Autodesk Inventor part; units mm, degrees
ref_plane "YZ Plane" through (0, 0, 0) normal (1, 0, 0) x (0, 1, 0)
ref_plane "XZ Plane" through (0, 0, 0) normal (0, 1, 0) x (-1, 0, 0)
ref_plane "XY Plane" through (0, 0, 0) normal (0, 0, 1) x (1, 0, 0)
sketch "Sketch1" plane through (0, 0, 0) normal (0, 1, 0) x (-1, 0, 0)
  line L0 (0, 0) -> (10, 0)
  line L1 (10, 0) -> (10, -12.7)
  line L2 (10, -12.7) -> (0, -12.7)
  line L3 (0, -12.7) -> (0, 0)
  dimension "d0" = 10
  dimension "d1" = 12.7
extrude "Extrusion1" add sketch "Sketch1" along normal blind 5.6
sketch "Sketch2" plane through (-10, 0, -12.7) normal (-1, 0, 0) x (0, 0, 1)
  line L0 (3.3, 4.8) -> (9.4, 4.8)
  line L1 (9.4, 4.8) -> (9.4, 0.8)
  line L2 (9.4, 0.8) -> (3.3, 0.8)
  line L3 (3.3, 0.8) -> (3.3, 4.8)
  line L4 (0, 0) -> (0, 5.6)
  point P0 (12.7, 0)
  point P1 (6.35, 4.8)
  point P2 (9.4, 2.8)
  dimension "d4" = 6.1
  dimension "d5" = 4
  dimension "d6" = 2.8
  dimension "d7" = 6.35
extrude "Extrusion2" cut sketch "Sketch2" against normal blind 1
sketch "Sketch3" plane through (-9, 0, -12.7) normal (-1, 0, 0) x (0, 0, 1)
  line L0 (5.8365, 4.7365) -> (9.3365, 4.7365)
  line L1 (9.3365, 4.7365) -> (9.3365, 0.8765)
  line L2 (9.3365, 0.8765) -> (5.8365, 0.8765)
  line L3 (5.8365, 0.8765) -> (5.8365, 4.7365)
  line L4 (9.4, 4.8) -> (9.4, 0.8)
  line L5 (3.3, 4.8) -> (9.4, 4.8)
  point P0 (12.7, 0)
  dimension "d10" = 3.5
  dimension "d11" = 3.86
  dimension "d12" = 0.0635
  dimension "d13" = 0.0635
extrude "Extrusion3" add sketch "Sketch3" along normal blind 5.72
properties part number "103-5007-EV"
Can you work these out from the model? Positions are in its coordinate system, mm. A direction names the side the tool comes from. Coordinates: 2 decimals unless noted, no trailing zeros. Order: outer loops, then holes, each group sorted by start corner. A loop starts at its lowest first (then second) coordinate and runs counter-clockwise, first axis right, second up.
1. I need wall thicknesses on line 1 (Y direction, x = -14, z = -6); line 2 (X direction, y = 3.9, z = -12); line 3 (Z direction, x = -11, y = 3.65). Which ranges of each line are inside material? Lowest first, please.
2. If we section it at D-D (x = -11): Please give me the cut outline in (y, z).
3. For faces 5 (the face through (-12, 4.736, -5)), 6 (the face through (0, 3, -6)), which set-ups out of +Z, -Z, +X, -X, +Y, -Y let a thin tool reach every point of the face, with its end or its side?
4. If we section it at C-C (z = -6): Please give me the cut outline in (x, y).
5. I'm going to push flat-ended pins straight in: pin 1 (0.5 mm diameter, centred on x = -9.5, y = 3.5, fed in from +Z); pin 2 (2 mm diameter, centred on x = -11.5, y = 3, fed in from +Z); pin 3 (1 mm diameter, centred on x = -12, z = -4.5, fed in from +Y); pin 4 (3 mm diameter, centred on y = 2.5, z = -10.5, fed in from -X). Where does each tip first touch, or does it pass through?
6. If we section it at A-A (x = -9.25): Please give me the cut outline in (y, z).
7. If we section it at B-B (y = 4.55): Please give me the cut outline in (x, z).
8. Thinking about a two-plate mould opening in Z: for faces 1 (the face through (-9, 3, -8)), 2 (the face through (-14.72, 3, -5)), 3 (the face through (-9.5, 2.8, -9.4)), 4 (the face through (-5, 3, 0)), which applies, +Z half, -Z half, draft (parallel to the pull), parting line (faces both ways), or undercut?
Entries:
1. line 1: y = 0.88 to 4.74
1. line 2: x = -10 to 0
1. line 3: z = -6.86 to -3.36
2. outline: (0.88, -6.86) - (4.74, -6.86) - (4.74, -3.36) - (0.88, -3.36) - close
3. face 5: -X
3. face 6: +Z, -Z, +X, +Y, -Y
4. outline: (-14.72, 0.88) - (-9, 0.88) - (-9, 0.8) - (-10, 0.8) - (-10, 0) - (0, 0) - (0, 5.6) - (-10, 5.6) - (-10, 4.8) - (-9, 4.8) - (-9, 4.74) - (-14.72, 4.74) - close
5. pin 1: stops at z = 0
5. pin 2: stops at z = -3.36
5. pin 3: stops at y = 4.74
5. pin 4: stops at x = -10
6. outline: (0, -12.7) - (5.6, -12.7) - (5.6, 0) - (0, 0) - close; (0.88, -6.86) - (4.74, -6.86) - (4.74, -3.36) - (0.88, -3.36) - close; hole (0.8, -9.4) - (4.8, -9.4) - (4.8, -3.3) - (0.8, -3.3) - close
7. outline: (-14.72, -6.86) - (-9, -6.86) - (-9, -9.4) - (-10, -9.4) - (-10, -12.7) - (0, -12.7) - (0, 0) - (-10, 0) - (-10, -3.3) - (-9, -3.3) - (-9, -3.36) - (-14.72, -3.36) - close
8. face 1: undercut
8. face 2: draft
8. face 3: undercut
8. face 4: +Z half
